Verification items for the finished model (mm, model axes). A direction names the side the tool comes from. Round coordinates to 2 decimals unless told otherwise and drop trailing zeros. Order: outer loops, then holes, each group sorted by start corner. A loop starts at its lowest first (then second) coordinate and runs counter-clockwise, first axis right, second up. Notation, with made-up numbers: (-2.75, 7) -> (43.25, 7) arc R24 ccw to (43.25, 28) -> close; hole circle Ø1 at (20.25, 69). An arc over 180 degrees is marked (long way). Return JSON: item names as keys, results as strings. Group by question number.
1) Section check C-C on z = -22. Enter the section's corners in (x, y), plus the area to 3 significant figures.
2) Section check A-A on z = -35. Enter the section's corners in (x, y), plus the area to 3 significant figures.
3) Section check B-B on y = 30. Enter the section's corners in (x, z), plus the area to 3 significant figures.
4) Scan lines: L1, parallel to Y at x = 2.75, z = -6; L2, parallel to X at y = 6, z = -48; L3, parallel to Y at x = 4.25, z = -52.5. Record each from-to range of solid material in increasing order.
5) Tool access check on faces 5 (the cylindrical face through (3.84, 45.24, -56.94)), 6 (the flat face through (8, 13.7, -46.2)), 7 (the flat face through (4, 4.8, -35.1)), 8 (the flat face through (4, 35, -52)). Record the directions out of +Z, -Z, +X, -X, +Y, -Y that give a thin tool (end or side, any length) a straight path to the whole face; none if there is none.
6) Depth check by flat-ended pin: pin 1 (0.5 mm diameter, centred on x = 3.5, z = -60.5, fed in from -Y); pin 2 (12.5 mm diameter, centred on y = 9.5, z = -32, fed in from +X); pin 3 (0.9 mm diameter, centred on x = 1, z = -35, fed in from +Y); pin 4 (1 mm diameter, centred on x = 1, y = 20.5, fed in from +Z). Enter the tip coordinate at first touch or a pass-through.
7) Section check D-D on z = -44.5. Enter the section's corners in (x, y), plus the area to 3 significant figures.
8) Draft check along X on faces 1 (the cylindrical face through (4.672, 5.07, -13.054)), 2 (the cylindrical face through (3.94, 28.1, -57.86)), 3 (the flat face through (0, 14, -30)), 4 (the flat face through (3, 3, -1)). Enter one of: pulls with the +X half, pulls with the -X half, needs draft (parallel to the pull), parting line crosses it, or undercut.
```python
from build123d import *

# Parameters (mm, degrees)
SKETCH1_W                   = 61
SKETCH1_H                   = 49
SKETCH1_R                   = 2.5
SKETCH1_R_2                 = 3
BOSS_EXTRUDE1_DEPTH         = 8
CUT_EXTRUDE2_REACH          = 80.651
SKETCH3_W                   = 4
SKETCH3_H                   = 29
FILLET2_R                   = 3
TAP_DRILL_FOR_M3_TAP1_D     = 2.5
TAP_DRILL_FOR_M3_TAP1_DEPTH = 10
TAP_DRILL_FOR_M3_TAP1_TIP   = 0.751075774
TAP_DRILL_FOR_M3_TAP2_D     = 2.5
TAP_DRILL_FOR_M3_TAP2_DEPTH = 8
TAP_DRILL_FOR_M3_TAP2_TIP   = 0.751075774
CUT_EXTRUDE3_DEPTH          = 8
CUT_EXTRUDE4_DEPTH          = 5
SKETCH14_R                  = 3
BOSS_EXTRUDE2_DEPTH         = 1
FILLET3_R                   = 5
FILLET4_R                   = 1.5


with BuildPart() as part:
    # Sketch1 → Boss-Extrude1 (new body)
    with BuildSketch(Plane(origin=(0, 0, 0), x_dir=(0, 0, -1), z_dir=(1, 0, 0))):
        with Locations((30.5, 24.5)):
            Rectangle(SKETCH1_W, SKETCH1_H)
        with Locations((6, 14.5)):
            Circle(SKETCH1_R, mode=Mode.SUBTRACT)
        with Locations((35, 8)):
            Circle(SKETCH1_R_2, mode=Mode.SUBTRACT)
    extrude(amount=BOSS_EXTRUDE1_DEPTH)

    # Sketch3 → Cut-Extrude2 (cut, up to next)
    with BuildSketch(Plane(origin=(8, 0, 0), x_dir=(0, 0, -1), z_dir=(1, 0, 0)), mode=Mode.PRIVATE) as cut_extrude2_sk1:
        with Locations((59, 14.5)):
            Rectangle(SKETCH3_W, SKETCH3_H)
    cut_extrude2_tool1 = extrude(cut_extrude2_sk1.sketch, amount=-CUT_EXTRUDE2_REACH, mode=Mode.PRIVATE) & part.part
    add(cut_extrude2_tool1.solids().sort_by_distance((8, 14.5, -59))[0], mode=Mode.SUBTRACT)

    # Fillet2
    fillet2_edges = [part.edges().sort_by_distance(p)[0] for p in [
        (4, 29, -57),
    ]]
    fillet(fillet2_edges, radius=FILLET2_R)

    # Tap Drill for M3 Tap1
    with Locations(Plane(origin=(0, 0, 0), x_dir=(-1, 0, 0), z_dir=(0, -1, 0))):
        with Locations((-4, 48), (-4, 12)):
            Hole(TAP_DRILL_FOR_M3_TAP1_D / 2, depth=TAP_DRILL_FOR_M3_TAP1_DEPTH)
            with Locations((0, 0, -(TAP_DRILL_FOR_M3_TAP1_DEPTH + TAP_DRILL_FOR_M3_TAP1_TIP / 2))):  # 118° drill point
                Cone(0, TAP_DRILL_FOR_M3_TAP1_D / 2, TAP_DRILL_FOR_M3_TAP1_TIP, mode=Mode.SUBTRACT)

    # Tap Drill for M3 Tap2
    with Locations(Plane(origin=(0, 0, -61), x_dir=(-1, 0, 0), z_dir=(0, 0, -1))):
        with Locations((-4, 44), (-4, 34)):
            Hole(TAP_DRILL_FOR_M3_TAP2_D / 2, depth=TAP_DRILL_FOR_M3_TAP2_DEPTH)
            with Locations((0, 0, -(TAP_DRILL_FOR_M3_TAP2_DEPTH + TAP_DRILL_FOR_M3_TAP2_TIP / 2))):  # 118° drill point
                Cone(0, TAP_DRILL_FOR_M3_TAP2_D / 2, TAP_DRILL_FOR_M3_TAP2_TIP, mode=Mode.SUBTRACT)

    # Sketch9 → Cut-Extrude3 (cut)
    with BuildSketch(Plane(origin=(8, 0, 0), x_dir=(0, 0, -1), z_dir=(1, 0, 0))):
        with BuildLine():
            Line((6, 20.5), (46, 20.5))
            ThreePointArc((46, 20.5), (50.242640687, 22.257359313), (52, 26.5))
            Line((52, 26.5), (52, 49))
            Line((52, 49), (0, 49))
            Line((0, 49), (0, 14.5))
            ThreePointArc((0, 14.5), (1.757359313, 18.742640687), (6, 20.5))
        make_face()
    extrude(amount=-CUT_EXTRUDE3_DEPTH, mode=Mode.SUBTRACT)

    # Sketch13 → Cut-Extrude4 (cut)
    with BuildSketch(Plane(origin=(8, 0, 0), x_dir=(0, 0, -1), z_dir=(1, 0, 0))):
        with BuildLine():
            Line((9.653047907, 19.259752199), (31.042531435, 2.843601785))
            ThreePointArc((31.042531435, 2.843601785), (36.300887291, 1.631507851), (40.662647671, 4.808695979))
            Line((40.662647671, 4.808695979), (51.227059389, 23.554180904))
            ThreePointArc((51.227059389, 23.554180904), (51.803548756, 24.97723218), (52, 26.5))
            Line((52, 26.5), (0, 26.5))
            Line((0, 26.5), (0, 14.5))
            ThreePointArc((0, 14.5), (3.346538811, 19.88137006), (9.653047907, 19.259752199))
        make_face()
        Polygon((0, 6), (3.5, 2.5), (3.5, 0), (0, 0), align=None)
    extrude(amount=-CUT_EXTRUDE4_DEPTH, mode=Mode.SUBTRACT)

    # Sketch14 → Boss-Extrude2 (add)
    with BuildSketch(Plane(origin=(3, 0, 0), x_dir=(0, 0, -1), z_dir=(1, 0, 0))):
        with BuildLine():
            Line((27.747742168, 5.372309694), (31.042531435, 2.843601785))
            ThreePointArc((31.042531435, 2.843601785), (36.300887291, 1.631507851), (40.662647671, 4.808695979))
            Line((40.662647671, 4.808695979), (42.701798604, 8.426964))
            ThreePointArc((42.701798604, 8.426964), (41.146254574, 7.684192991), (39.919256736, 8.894937519))
            ThreePointArc((39.919256736, 8.894937519), (33.999317468, 12.898840115), (30.123849342, 6.894036726))
            ThreePointArc((30.123849342, 6.894036726), (29.469968742, 5.299086519), (27.747742168, 5.372309694))
        make_face()
        with Locations((35, 8)):
            Circle(SKETCH14_R, mode=Mode.SUBTRACT)
    extrude(amount=BOSS_EXTRUDE2_DEPTH)

    # Fillet3
    fillet3_edges = [part.edges().sort_by_distance(p)[0] for p in [
        (4, 49, -52),
    ]]
    fillet(fillet3_edges, radius=FILLET3_R)

    # Fillet4
    fillet4_edges = [part.edges().sort_by_distance(p)[0] for p in [
        (5.5, 6, 0),
        (5.5, 2.5, -3.5),
    ]]
    fillet(fillet4_edges, radius=FILLET4_R)


solid = part.part
```
Check result:
{
 "1": {"outline": "(0, 0) -> (8, 0) -> (8, 9.78) -> (3, 9.78) -> (3, 20.5) -> (0, 20.5) -> close", "area": "110 mm^2"},
 "2": {"outline": "(0, 0) -> (8, 0) -> (8, 1.5) -> (4, 1.5) -> (4, 5) -> (0, 5) -> close; (0, 11) -> (4, 11) -> (4, 13) -> (3, 13) -> (3, 20.5) -> (0, 20.5) -> close", "area": "56.5 mm^2"},
 "3": {"outline": "(0, -61) -> (8, -61) -> (8, -52) -> (0, -52) -> close", "area": "72.0 mm^2"},
 "4": {"L1": "0 to 12, 17 to 20.5", "L2": "0 to 2.75, 5.25 to 8", "L3": "0 to 33.67, 34.33 to 43.67, 44.33 to 46.18"},
 "5": {"face 5": "-Z", "face 6": "+Z, -Z, +X, +Y, -Y", "face 7": "+X, +Y", "face 8": "+Z, +X, -X, +Y"},
 "6": {"pin 1": "y = 29", "pin 2": "x = 8", "pin 3": "y = 20.5", "pin 4": "z = -3.6"},
 "7": {"outline": "(0, 0) -> (8, 0) -> (8, 11.62) -> (3, 11.62) -> (3, 20.5) -> (0, 20.5) -> close", "area": "120 mm^2"},
 "8": {"face 1": "undercut", "face 2": "needs draft", "face 3": "pulls with the -X half", "face 4": "pulls with the +X half"}
}
